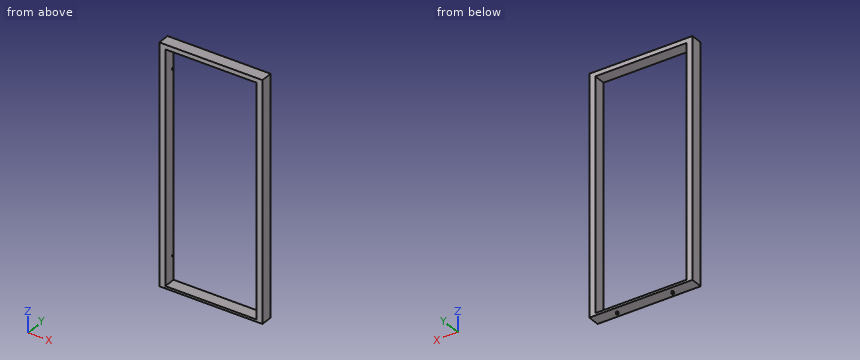
```python
from build123d import *

# Parameters (mm, degrees)
F0_W     = 50
F0_H     = 1942
F0_W_2   = 865
F0_H_2   = 20
F1_DEPTH = 50
F3_R     = 10
F4_DEPTH = 15
F6_R     = 6
F7_DEPTH = 4


with BuildPart() as f1:
    # F0 (on Front) → F1 (new body, symmetric)
    with BuildSketch(Plane.XZ):
        with Locations((-407.5, 0)):
            Rectangle(F0_W, F0_H)
        Polygon((432.5, 990), (-432.5, 990), (-432.5, 971), (-382.5, 971), (382.5, 971), (432.5, 971), align=None)
        with Locations((0, 1000)):
            Rectangle(F0_W_2, F0_H_2)
        with Locations((407.5, 0)):
            Rectangle(F0_W, F0_H)
        Polygon((-382.5, -971), (-432.5, -971), (-432.5, -990), (432.5, -990), (432.5, -971), (382.5, -971), align=None)
    extrude(amount=F1_DEPTH, both=True)

    # F3 (on offset) → F4 (join)
    with BuildSketch(Plane.XY.offset(-990)):
        with Locations((-232.5, 0)):
            Circle(F3_R)
        with Locations((232.5, 0)):
            Circle(F3_R)
    extrude(amount=-F4_DEPTH)

    # F6 (on offset) → F7 (join)
    with BuildSketch(Plane.YZ.offset(-382.5)):
        with Locations((35, 766)):
            Circle(F6_R)
        with Locations((35, -766)):
            Circle(F6_R)
    extrude(amount=F7_DEPTH)


solid = f1.part
```
Could you check a few things on this model? Use its own coordinates, in mm. Coordinates: 2 decimals unless noted, no trailing zeros. Loops run counter-clockwise (first coordinate to the right, second up) from the corner with the lowest first, then second, coordinate; pieces in that order, holes last.
1) Please list where these lines run through material, in increasing order: line 1 along X through (y, z) = (-39.5, 89); line 2 along Z through (x, y) = (-303, -7).
Reported:
line 1: x = -432.5 to -382.5, 382.5 to 432.5
line 2: z = -990 to -971, 971 to 1010
2) Imagine slicing it at B-B (x = 321). List the corners of the cut face in (y, z) for me.
Reported:
outline: (-50, -990) - (50, -990) - (50, -971) - (-50, -971) - close; (-50, 971) - (50, 971) - (50, 1010) - (-50, 1010) - close
3) Will this pin go through, and if not, where does the flat tip stop? pin 1 Ø6 at (x, y) = (204.5, -33) entering from -Z.
Reported:
pin 1: stops at z = -990
4) Imagine slicing it at A-A (z = 127). List the corners of the cut face in (x, y) for me.
Reported:
outline: (-432.5, -50) - (-382.5, -50) - (-382.5, 50) - (-432.5, 50) - close; (382.5, -50) - (432.5, -50) - (432.5, 50) - (382.5, 50) - close
